For this review, take the finished solid that the model builds, in its own axes (mm). Face numbers are marked on the shaded views. A direction names the side the tool comes from. Coordinates: 2 decimals unless noted, no trailing zeros. Loops run counter-clockwise (first coordinate to the right, second up) from the corner with the lowest first, then second, coordinate; pieces in that order, holes last.
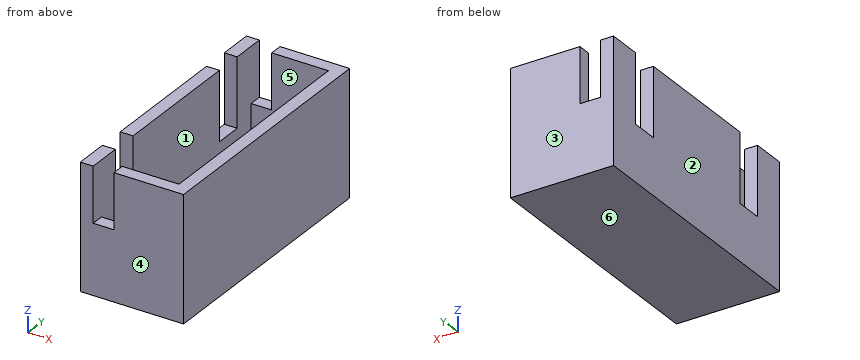
```python
from build123d import *

# Parameters (mm, degrees)
BOX001_W        = 4.5
BOX001_H        = 13.5
BOX001_DEPTH    = 6.5
THICKNESS_T     = 0.75
SKETCH002_W     = 1.6
SKETCH002_H     = 4
POCKET001_DEPTH = 0.75
SKETCH003_W     = 1.2
SKETCH003_H     = 3.2
POCKET002_DEPTH = 15.001


with BuildPart() as part:
    # Box001 → Box001 (new body)
    with BuildSketch(Plane(origin=(-8.25, -13.2, 2.25), x_dir=(1, 0, 0), z_dir=(0, 0, 1))):
        with Locations((2.25, 6.75)):
            Rectangle(BOX001_W, BOX001_H)
    extrude(amount=BOX001_DEPTH)

    # Thickness
    thickness_openings = [part.faces().sort_by_distance(p)[0] for p in [
        (-6, -6.45, 8.75),
    ]]
    offset(amount=THICKNESS_T, openings=thickness_openings, kind=Kind.INTERSECTION)

    # Sketch002 → Pocket001 (cut)
    with BuildSketch(Plane(origin=(-9, 0, 0), x_dir=(0, -1, 0), z_dir=(-1, 0, 0))):
        with Locations((1.75, 6.75)):
            Rectangle(SKETCH002_W, SKETCH002_H)
        with Locations((11.15, 6.75)):
            Rectangle(SKETCH002_W, SKETCH002_H)
    extrude(amount=-POCKET001_DEPTH, mode=Mode.SUBTRACT)

    # Sketch003 → Pocket002 (cut, through all)
    with BuildSketch(Plane.XZ.offset(13.95)):
        with Locations((-7.65, 7.15)):
            Rectangle(SKETCH003_W, SKETCH003_H)
    extrude(amount=-POCKET002_DEPTH, mode=Mode.SUBTRACT)


solid = part.part
```
Q1. The part is to be moulded in two halves that separate along Y. For the marked faces 3, 4, 5 and 6, say which applies: +Y half, -Y half, draft (parallel to the pull), parting line (faces both ways), or undercut.
Q2. For pin 1 Ø0.8 at (x, y) = (-9, -11) entering from +Z; pin 2 Ø1.3 at (x, y) = (-5.5, -6) entering from +Z, all flat-tipped, find the tip position at first contact; note any pin that passes through.
Q3. Wall thickness on probe 1 along X at (y, z) = (-7, 4.75); probe 2 along Y at (x, z) = (-4.75, 7.5): over which ranges is each line inside the solid? List them lowest first.
Q4. Consider section C-C (x = -6.85). State the section outline as (y, z) points.
Q5. Consider section D-D (z = 7). State the section outline as (x, y) points.
Q6. Consider section B-B (y = -1.5). State the section outline as (x, z) points.
Q7. Machinability: for the marked faces 1 and 2, which of the approach directions +Z, -Z, +X, -X, +Y, -Y give a long, thin tool a straight path to every point of the face, cutting with its end or side? Answer none if there is none.
Q8. Consider section A-A (z = 2.5). State the section outline as (x, y) points.
Model answer:
1. face 3: +Y half
1. face 4: -Y half
1. face 5: undercut
1. face 6: draft
2. pin 1: stops at z = 4.75
2. pin 2: stops at z = 2.25
3. probe 1: x = -9 to -8.25, -3.75 to -3
3. probe 2: y = -13.95 to -13.2, 0.3 to 1.05
4. outline: (-13.95, 1.5) - (1.05, 1.5) - (1.05, 8.75) - (0.3, 8.75) - (0.3, 2.25) - (-13.2, 2.25) - (-13.2, 8.75) - (-13.95, 8.75) - close
5. outline: (-9, -13.95) - (-8.25, -13.95) - (-8.25, -11.95) - (-9, -11.95) - close; (-9, -10.35) - (-8.25, -10.35) - (-8.25, -2.55) - (-9, -2.55) - close; (-9, -0.95) - (-8.25, -0.95) - (-8.25, 1.05) - (-9, 1.05) - close; (-7.05, -13.95) - (-3, -13.95) - (-3, 1.05) - (-7.05, 1.05) - (-7.05, 0.3) - (-3.75, 0.3) - (-3.75, -13.2) - (-7.05, -13.2) - close
6. outline: (-9, 1.5) - (-3, 1.5) - (-3, 8.75) - (-3.75, 8.75) - (-3.75, 2.25) - (-8.25, 2.25) - (-8.25, 4.75) - (-9, 4.75) - close
7. face 1: +Z
7. face 2: +Z, -Z, -X, +Y, -Y
8. outline: (-9, -13.95) - (-3, -13.95) - (-3, 1.05) - (-9, 1.05) - close; hole (-8.25, -13.2) - (-3.75, -13.2) - (-3.75, 0.3) - (-8.25, 0.3) - close
